The model under review builds one solid part; all positions refer to its coordinate system, in mm. Face numbers are marked on the shaded views. A direction names the side the tool comes from. Round coordinates to 2 decimals unless told otherwise and drop trailing zeros. Write each loop counter-clockwise with the first axis right and the second up, starting at its lowest first coordinate (ties: lowest second). Pieces come first, ordered by that corner, then holes. Notation, with made-up numbers: M -21.5,47.5 L 22.5,47.5 A24 ccw 22.5,70.5 Z; hole C 81.25,1.25 d4. An arc over 180 degrees is marked long. Write item = value, one per line. Start each with the question number.
Item 1: Take a section at D-D, the plane z = 4. Give the boundary of the cut face in (x, y).
Item 2: Take a section at C-C, the plane z = 10. Give the boundary of the cut face in (x, y), plus the area to 3 significant figures.
Item 3: For pin 1 Ø8 at (x, y) = (6, 3.5) entering from -Z; pin 2 Ø1.4 at (x, y) = (0, 0) entering from +Z; pin 3 Ø1.5 at (y, z) = (3.5, 9) entering from +X; pin 4 Ø4 at (y, z) = (2, 21.5) entering from +X, all flat-tipped, find the tip position at first contact; note any pin that passes through.
Item 4: To check wall thickness, follow line 1 along Y through (x, z) = (0, 19.75); line 2 along Z through (x, y) = (-6.75, -2.75); line 3 along Y through (x, z) = (0.5, 20.75). State the ranges of each line that lie inside material, in increasing order.
Item 5: Tool access review of the marked faces 1 and 2: name each direction out of +Z, -Z, +X, -X, +Y, -Y from which nothing blocks a thin tool from reaching the whole face with its end or side.
Item 6: Take a section at A-A, the plane y = 0. Give the boundary of the cut face in (x, z).
from build123d import *

# Parameters (mm, degrees)
F2_R     = 0.5
F3_SIZE2 = 2
F3_SIZE  = 6
F4_R     = 0.5
F6_D     = 2.3
F7_R     = 0.5


with BuildPart() as f1:
    # F0 (on Front) → F1 (revolve)
    with BuildSketch(Plane.XZ):
        Polygon((8, 27.8), (0, 27.8), (0, 0), (5.75, 0), (5.75, 26), (8, 26), align=None)
    revolve(axis=Axis((0, 0, 13.9), (0, 0, -1)))

    # F2
    f2_edges = [f1.edges().sort_by_distance(p)[0] for p in [
        (-5.75, 0, 26),
    ]]
    fillet(f2_edges, radius=F2_R)

    # F3
    f3_edges = [f1.edges().sort_by_distance(p)[0] for p in [
        (-5.75, 0, 0),
    ]]
    chamfer(f3_edges, length=F3_SIZE, length2=F3_SIZE2)

    # F4
    f4_edges = [f1.edges().sort_by_distance(p)[0] for p in [
        (-3.75, 0, 0),
    ]]
    fillet(f4_edges, radius=F4_R)

    # F6 (through all)
    with Locations(Plane.XY.offset(27.8)):
        with Locations((0, 0)):
            Hole(F6_D / 2)

    # F7
    f7_edges = [f1.edges().sort_by_distance(p)[0] for p in [
        (-8, 0, 26),
    ]]
    fillet(f7_edges, radius=F7_R)


solid = f1.part
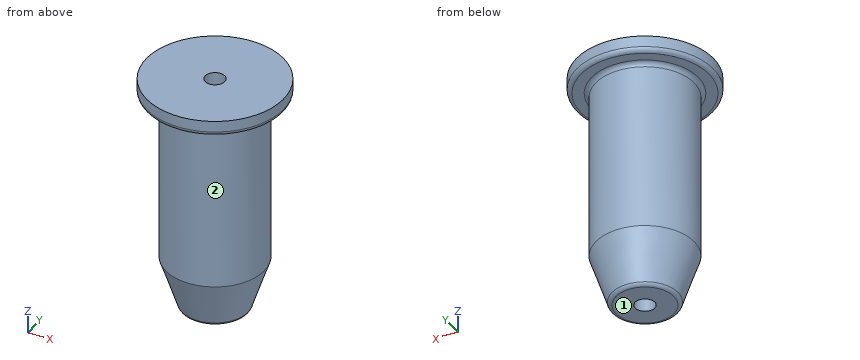
Response values:
q1.outline = C 0,0 d10.17; hole C 0,0 d2.3
q2.outline = C 0,0 d11.5; hole C 0,0 d2.3
q2.area = 99.7 mm2
q3.pin_1 = 0
q3.pin_2 = through
q3.pin_3 = 5.05
q3.pin_4 = 5.75
q4.line_1 = -5.75 to -1.15, 1.15 to 5.75
q4.line_2 = 26 to 27.8
q4.line_3 = -5.73 to -1.04, 1.04 to 5.73
q5.face_1 = -Z, +X, -X, +Y, -Y
q5.face_2 = -Z
q6.outline = M -8,26.5 A0.5 ccw -7.5,26 L -6.25,26 A0.5 cw -5.75,25.5 L -5.75,6 L -3.86,0.34 A0.5 ccw -3.39,0 L -1.15,0 L -1.15,27.8 L -8,27.8 Z; M 1.15,0 L 3.39,0 A0.5 ccw 3.86,0.34 L 5.75,6 L 5.75,25.5 A0.5 cw 6.25,26 L 7.5,26 A0.5 ccw 8,26.5 L 8,27.8 L 1.15,27.8 Z
